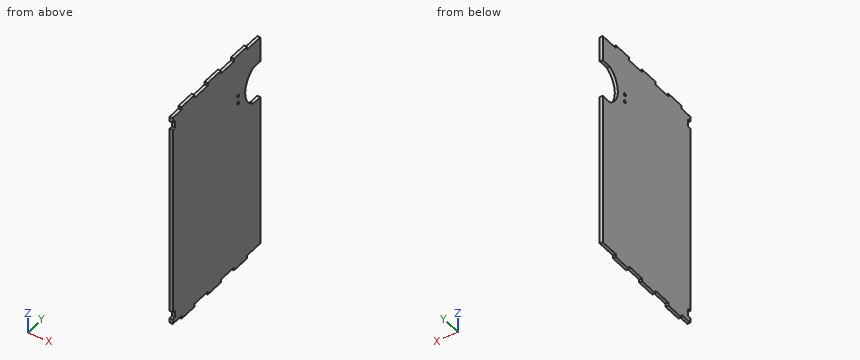
from build123d import *

# Parameters (mm, degrees)
SKETCH1_W            = 450
SKETCH1_H            = 250
BOSS_EXTRUDE1_DEPTH  = 6
SKETCH2_W            = 6
SKETCH2_H            = 37.5
CUT_EXTRUDE1_DEPTH   = 515.816472153
LPATTERN1_COUNT      = 4
LPATTERN1_PITCH      = 75
LPATTERN1_COUNT_DIR2 = 2
LPATTERN1_PITCH_DIR2 = 444
SKETCH3_W            = 15
SKETCH3_H            = 6
CUT_EXTRUDE2_DEPTH   = 515.816472153
LPATTERN2_COUNT      = 2
LPATTERN2_PITCH      = 403
SKETCH4_R            = 3
CUT_EXTRUDE3_DEPTH   = 10


with BuildPart() as part:
    # Sketch1 → Boss-Extrude1 (new body)
    with BuildSketch(Plane(origin=(0, 0, 0), x_dir=(0, 0, -1), z_dir=(1, 0, 0))):
        with Locations((-225, 125)):
            Rectangle(SKETCH1_W, SKETCH1_H)
    extrude(amount=BOSS_EXTRUDE1_DEPTH)

    # Sketch2 → Cut-Extrude1 (cut, through all)
    with BuildSketch(Plane(origin=(6, 0, 0), x_dir=(0, 0, -1), z_dir=(1, 0, 0))):
        with Locations((-447, 231.25)):
            Rectangle(SKETCH2_W, SKETCH2_H)
    cut_extrude1 = extrude(amount=-CUT_EXTRUDE1_DEPTH, mode=Mode.SUBTRACT)

    # LPattern1: Cut-Extrude1 4 × 2
    with Locations(*[(0, -i * LPATTERN1_PITCH, -j * LPATTERN1_PITCH_DIR2) for i in range(LPATTERN1_COUNT) for j in range(LPATTERN1_COUNT_DIR2) if (i, j) != (0, 0)]):
        add(cut_extrude1, mode=Mode.SUBTRACT)

    # Sketch3 → Cut-Extrude2 (cut, through all)
    with BuildSketch(Plane(origin=(6, 0, 0), x_dir=(0, 0, -1), z_dir=(1, 0, 0))):
        with Locations((-426.5, 3)):
            Rectangle(SKETCH3_W, SKETCH3_H)
    cut_extrude2 = extrude(amount=-CUT_EXTRUDE2_DEPTH, mode=Mode.SUBTRACT)

    # LPattern2: Cut-Extrude2 ×2
    with Locations(*[(0, 0, -i * LPATTERN2_PITCH) for i in range(1, LPATTERN2_COUNT)]):
        add(cut_extrude2, mode=Mode.SUBTRACT)

    # Sketch4 → Cut-Extrude3 (cut)
    with BuildSketch(Plane(origin=(6, 0, 0), x_dir=(0, 0, -1), z_dir=(1, 0, 0))):
        with Locations((-362.5, 187)):
            Circle(SKETCH4_R)
        with Locations((-347.5, 187)):
            Circle(SKETCH4_R)
        with BuildLine():
            Line((-393.065732621, 230), (-393.065732621, 250))
            Line((-393.065732621, 250), (-316.934267379, 250))
            Line((-316.934267379, 250), (-316.934267379, 230))
            ThreePointArc((-316.934267379, 230), (-355, 207), (-393.065732621, 230))
        make_face()
    extrude(amount=-CUT_EXTRUDE3_DEPTH, mode=Mode.SUBTRACT)


solid = part.part
Build history of the part. All positions in model axes, mm. Round coordinates to 2 decimals unless told otherwise and drop trailing zeros. Write each loop counter-clockwise with the first axis right and the second up, starting at its lowest first coordinate (ties: lowest second). Pieces come first, ordered by that corner, then holes. Notation, with made-up numbers: M 66.5,71.5 L 73.5,71.5 A32 cw 73.5,99.5 Z; hole C 80.5,49 d5. An arc over 180 degrees is marked long. Answer in a Markdown table with one row per item.
1. Flat gauge pins, fed straight in: P1, Ø5.5, axis at y = 187, z = 347.5, coming from the -X side; P2, Ø2, axis at x = 4.5, y = 140, coming from the -Z side; P3, Ø1.8, axis at x = 3, z = 2, coming from the +Y side; P4, Ø1.8, axis at x = 3, y = 3.5, coming from the +Z side. Where does each tip first touch, or does it go through?
Geometry check:
| item | result |
|---|---|
| P1 | through |
| P2 | z = 6 |
| P3 | y = 212.5 |
| P4 | z = 444 |
2. Probe L1, parallel to Z at x = 1.7, y = 187; L2, parallel to Y at x = 4.9, z = 428.5; L3, parallel to Z at x = 0.5, y = 24.5. List the from-to ranges inside material, lowest first. Write a range as [from, to].
Geometry check:
| item | result |
|---|---|
| L1 | [0, 344.5], [350.5, 359.5], [365.5, 450] |
| L2 | [6, 250] |
| L3 | [6, 444] |
3. Saw through at B-B (x = 4.7). State how many separate pieces and enclosed holes the cut face has, and give its area (3 significant figures).
Geometry check:
| item | result |
|---|---|
| separate pieces | 1 |
| enclosed holes | 2 |
| area | 108,000 mm2 |
4. Saw through at A-A (y = 164.5). List the corners of the cut face in (x, z), and give its area (3 significant figures).
Geometry check:
| item | result |
|---|---|
| outline | M 0,6 L 6,6 L 6,444 L 0,444 Z |
| area | 2,630 mm2 |
